Work out the finished part from the listing and answer in its coordinate system (mm). Coordinates: 2 decimals unless noted, no trailing zeros. Write each loop counter-clockwise with the first axis right and the second up, starting at its lowest first coordinate (ties: lowest second). Pieces come first, ordered by that corner, then holes. Notation, with made-up numbers: (49.25, 46.25) - (85.25, 46.25) arc R21 ccw to (85.25, 52.25) - close; hole circle Ø5 at (-19, 64.5). An arc over 180 degrees is marked (long way). Answer as a JSON object with one key per item and string values. Group by question number.
from build123d import *

# Parameters (mm, degrees)
F1_DEPTH = 100


with BuildPart() as f1:
    # F0 (on Top) → F1 (new body)
    with BuildSketch(Plane.XY):
        with BuildLine():
            Line((20.24916, 30.557973), (18.683154, 32.452531))
            ThreePointArc((18.683154, 32.452531), (-0.526402, 34.65267), (-19.74347, 32.519136))
            Line((-19.74347, 32.519136), (-20.249992, 30.505758))
            ThreePointArc((-20.249992, 30.505758), (-18.414901, 14.379255), (-12.91545, -0.89123))
            Line((-12.91545, -0.89123), (-11.125, -2))
            Line((-11.125, -2), (0, -2))
            Line((0, -2), (11.125, -2))
            Line((11.125, -2), (12.89157, -0.937672))
            ThreePointArc((12.89157, -0.937672), (18.617034, 14.332035), (20.24916, 30.557973))
        make_face()
        with BuildLine():
            Line((11.125, 0), (0, 0))
            Line((0, 0), (-11.125, 0))
            ThreePointArc((-11.125, 0), (-16.501317, 14.980406), (-18.248473, 30.800166))
            ThreePointArc((-18.248473, 30.800166), (0.017215, 32.649949), (18.250002, 30.499932))
            ThreePointArc((18.250002, 30.499932), (16.669461, 14.786966), (11.125, 0))
        make_face(mode=Mode.SUBTRACT)
        with BuildLine():
            Line((-11.125, 0), (0, 0))
            Line((0, 0), (11.125, 0))
            ThreePointArc((11.125, 0), (16.669461, 14.786966), (18.250002, 30.499932))
            ThreePointArc((18.250002, 30.499932), (0.017215, 32.649949), (-18.248473, 30.800166))
            ThreePointArc((-18.248473, 30.800166), (-16.501317, 14.980406), (-11.125, 0))
        make_face()
    extrude(amount=F1_DEPTH)


solid = f1.part
Q1. Section A-A on z = 25.5 is taken. Determine the outline of the cut face in (x, y) (3 decimals).
Q2. Section C-C on y = 20 is taken. Determine the outline of the cut face in (x, z).
Q3. Section B-B on y = 7.5 is taken. Determine the outline of the cut face in (x, z), plus the area to 3 significant figures.
Q4. Consider L1, parallel to Y at x = 0, z = 54; L2, parallel to X at y = 29, z = 7.5; L3, parallel to Y at x = 4.5, z = 55. Determine where each line is inside the solid, lowest interval first. Write a range as from..to.
Q5. For a pull along Z with two mould halves and no side action, classify faces 1 (the face through (0, 17, 0)), 2 (the face through (0, 17, 100)), 3 (the face through (19.48, 31.49, 49.3)) as +Z half, -Z half, draft (parallel to the pull), parting line (faces both ways), or undercut.
Q6. Flat-ended cylindrical pins translate along their axes: pin 1 Ø2 at (y, z) = (4, 88.5) entering from +X; pin 2 Ø2 at (y, z) = (14, 24) entering from -X; pin 3 Ø5 at (x, y) = (-6, 25) entering from -Z. Find the tip coordinate at first contact, or state that the pin passes through.
Numbers:
{
 "1": {"outline": "(-20.25, 30.506) arc R70.005 ccw to (-12.915, -0.891) - (-11.125, -2) - (11.125, -2) - (12.892, -0.938) arc R63.267 ccw to (20.249, 30.558) - (18.683, 32.453) arc R86.266 ccw to (-19.743, 32.519) - close"},
 "2": {"outline": "(-19.49, 0) - (19.67, 0) - (19.67, 100) - (-19.49, 100) - close"},
 "3": {"outline": "(-16.43, 0) - (16.61, 0) - (16.61, 100) - (-16.43, 100) - close", "area": "3,300 mm²"},
 "4": {"L1": "y = -2..34.65", "L2": "x = -20.24..20.28", "L3": "y = -2..34.5"},
 "5": {"face 1": "-Z half", "face 2": "+Z half", "face 3": "draft"},
 "6": {"pin 1": "stops at x = 15.66", "pin 2": "stops at x = -18.56", "pin 3": "stops at z = 0"}
}
